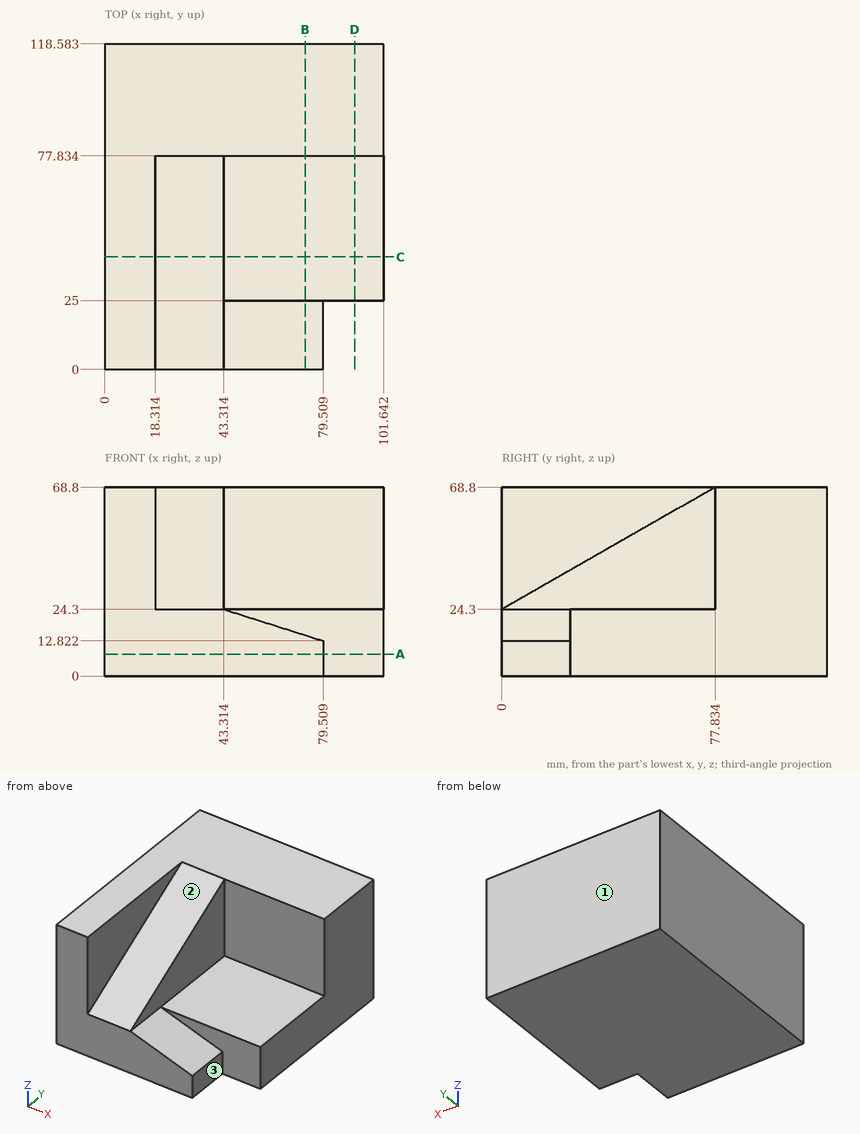
The drawing under review shows one solid part. Ordinate dimensions are in mm from its lowest x, y, z. A direction names the side the tool comes from. Round coordinates to 2 decimals unless told otherwise and drop trailing zeros. Write each loop counter-clockwise with the first axis right and the second up, starting at its lowest first coordinate (ties: lowest second). Pieces come first, ordered by that corner, then holes. Notation, with made-up numbers: (52.25, 2.5) - (107.25, 2.5) arc R22 cw to (107.25, 39.5) - close; hole circle Ø6 at (82.25, -10). An arc over 180 degrees is marked (long way). Use a Markdown table: item, result. Add a question column.
1. Wall thickness on probe 1 along X at (y, z) = (31, 62); probe 2 along Y at (x, z) = (85, 46.5) (1 decimal); probe 3 along X at (y, z) = (76.5, 33): over which ranges is each line inside the solid? List them lowest first.
2. We need section C-C (y = 41). State the section outline as (x, z) points.
3. For the marked faces 1, 2 and 3, list the 3-axis set-ups (+Z, -Z, +X, -X, +Y, -Y) from which the entire face can be reached by the end or side of a thin tool; tool diameter is ignored.
4. We need section B-B (x = 73). State the section outline as (y, z) points (1 decimal).
5. Clearance check with flat-ended pins moving along their axes: pin 1 (1 mm diameter, centred on x = 82, y = 52, fed in from +Z); pin 2 (10 mm diameter, centred on x = 16.5, y = 101, fed in from -Z); pin 3 (22 mm diameter, centred on y = 47, z = 54, fed in from +X); pin 4 (6.5 mm diameter, centred on y = 10.5, z = 9.5, fed in from +X). State where each tip first meets the part, or that it passes through.
6. We need section D-D (x = 91). State the section outline as (y, z) points (1 decimal).
7. We need section A-A (z = 8). State the section outline as (x, y) points, then the cut area to 3 significant figures.
Output:
| question | item | result |
|---|---|---|
| 1 | probe 1 | x = 0 to 18.31 |
| 1 | probe 2 | y = 77.8 to 118.6 |
| 1 | probe 3 | x = 0 to 43.31 |
| 2 | outline | (0, 0) - (101.64, 0) - (101.64, 24.3) - (43.31, 24.3) - (43.31, 47.74) - (18.31, 47.74) - (18.31, 68.8) - (0, 68.8) - close |
| 3 | face 1 | +Z, -Z, +X, -X, +Y |
| 3 | face 2 | +Z, +X, -Y |
| 3 | face 3 | +Z, -Z, +X, -Y |
| 4 | outline | (0, 0) - (118.6, 0) - (118.6, 68.8) - (77.8, 68.8) - (77.8, 24.3) - (25, 24.3) - (25, 14.9) - (0, 14.9) - close |
| 5 | pin 1 | stops at z = 24.3 |
| 5 | pin 2 | stops at z = 0 |
| 5 | pin 3 | stops at x = 43.31 |
| 5 | pin 4 | stops at x = 79.51 |
| 6 | outline | (25, 0) - (118.6, 0) - (118.6, 68.8) - (77.8, 68.8) - (77.8, 24.3) - (25, 24.3) - close |
| 7 | outline | (0, 0) - (79.51, 0) - (79.51, 25) - (101.64, 25) - (101.64, 118.58) - (0, 118.58) - close |
| 7 | area | 11,500 mm2 |
